Work out the finished part from the listing and answer in its coordinate system (mm). A direction names the side the tool comes from. Round coordinates to 2 decimals unless told otherwise and drop trailing zeros. Loops run counter-clockwise (first coordinate to the right, second up) from the corner with the lowest first, then second, coordinate; pieces in that order, holes last. Notation, with made-up numbers: M 8,11 L 57,11 A22 cw 57,41 Z; hole C 53.5,-9.5 d8. An arc over 180 degrees is marked long. One line per item, written item: value.
```python
from build123d import *

# Parameters (mm, degrees)
ESQUISSE1_W      = 31.5
ESQUISSE1_H      = 19
EXTRUSION1_DEPTH = 3
EXTRUSION2_DEPTH = 5


with BuildPart() as part:
    # Esquisse1 → Extrusion1 (new body)
    with BuildSketch(Plane.XY):
        with Locations((-6.993175074, -6.195994065)):
            Rectangle(ESQUISSE1_W, ESQUISSE1_H)
    extrude(amount=-EXTRUSION1_DEPTH)

    # Esquisse2 → Extrusion2 (add, symmetric)
    with BuildSketch(Plane(origin=(0, -6.445994065, 0), x_dir=(-1, 0, 0), z_dir=(0, 1, 0))):
        with BuildLine():
            Line((-0.683946914, 1.503708235), (-1.522862282, 2.753870501))
            Line((-1.522862282, 2.753870501), (-0.951110198, 2.753870501))
            Line((-0.951110198, 2.753870501), (-1.764464322, 4.339195483))
            Line((-1.764464322, 4.339195483), (-1.070373593, 4.339195483))
            Line((-1.070373593, 4.339195483), (-1.522862282, 6.137827556))
            Line((-1.522862282, 6.137827556), (-0.919586302, 6.039619438))
            Line((-0.919586302, 6.039619438), (-0.919586302, 7.896542483))
            Line((-0.919586302, 7.896542483), (-0.491311221, 7.750686861))
            Line((-0.491311221, 7.750686861), (-0.194631359, 9.573141446))
            Line((-0.194631359, 9.573141446), (0.23155106, 9.427998511))
            Line((0.23155106, 9.427998511), (0.646902561, 11.526197473))
            Line((0.646902561, 11.526197473), (-0.919586302, 12.794183433))
            ThreePointArc((-0.919586302, 12.794183433), (-1.739109574, 14.422451612), (0.024155253, 13.960095898))
            Line((0.024155253, 13.960095898), (1.735137514, 12.575150538))
            Line((1.735137514, 12.575150538), (3.580381554, 13.110240468))
            ThreePointArc((3.580381554, 13.110240468), (6.259156873, 14.419297059), (9.196563315, 14.930286061))
            ThreePointArc((9.196563315, 14.930286061), (16.439211341, 8.707680897), (11.226331582, 0.70751527))
            ThreePointArc((11.226331582, 0.70751527), (10.958201165, 0.354142581), (11.225313893, 0))
            Line((11.225313893, 0), (3.908893256, 0))
            ThreePointArc((3.908893256, 0), (4.942460115, 0.812425826), (4.628744056, 2.089092739))
            ThreePointArc((4.628744056, 2.089092739), (2.440830828, 5.172896926), (2.103130606, 8.938898932))
            ThreePointArc((2.103130606, 8.938898932), (2.971882266, 9.547397538), (3.580380872, 8.678645878))
            ThreePointArc((3.580380872, 8.678645878), (12.939531774, 3.276526542), (9.243174696, 13.431010442))
            ThreePointArc((9.243174696, 13.431010442), (1.988346124, 9.431080483), (0.985709709, 1.207535171))
            ThreePointArc((0.985709709, 1.207535171), (0.089542016, 1.009824881), (-0.683946914, 1.503708235))
        make_face()
        with BuildLine():
            Line((0.024155253, 9.573141446), (-0.573596034, 9.77671478))
            Line((-0.573596034, 9.77671478), (-3.903205639, 0))
            Line((-3.903205639, 0), (-5.477057205, 0))
            Line((-5.477057205, 0), (-2.145067788, 9.78370261))
            Line((-2.145067788, 9.78370261), (-5.43013268, 10.902481655))
            ThreePointArc((-5.43013268, 10.902481655), (-6.770419213, 12.151238044), (-4.946559165, 12.322395968))
            Line((-4.946559165, 12.322395968), (-0.453501716, 10.7922166))
            Line((-0.453501716, 10.7922166), (0.024155253, 9.573141446))
        make_face()
    extrude(amount=EXTRUSION2_DEPTH, both=True)


solid = part.part
```
1) Find section B-B (z = 6.75). Give the vertices of the cut face in (x, y).
Check values:
outline: M -16.45,-11.45 L -14.92,-11.45 L -14.92,-1.45 L -16.45,-1.45 Z; M -3.57,-11.45 L -2.05,-11.45 L -2.05,-1.45 L -3.57,-1.45 Z; M -0.75,-11.45 L 0.92,-11.45 L 0.92,-1.45 L -0.75,-1.45 Z; M 1.6,-11.45 L 3.18,-11.45 L 3.18,-1.45 L 1.6,-1.45 Z
2) Each of these flat-tipped pins is pushed along its axis until it touches: pin 1 (1.5 mm diameter, centred on x = -0.5, z = 3.5, fed in from +Y); pin 2 (4 mm diameter, centred on y = -5.5, z = 3, fed in from -X); pin 3 (10 mm diameter, centred on x = -17, y = -5, fed in from +Z). Where does it stop, or does it pass through?
Check values:
pin 1: y = -1.45
pin 2: x = -16
pin 3: z = 14.39
3) Find section C-C (x = -8). Give the vertices of the cut face in (y, z).
Check values:
outline: M -15.7,-3 L 3.3,-3 L 3.3,0 L -1.45,0 L -1.45,2.07 L -11.45,2.07 L -11.45,0 L -15.7,0 Z; M -11.45,13.31 L -1.45,13.31 L -1.45,14.82 L -11.45,14.82 Z
4) The mould has two halves that part along X. Classify faces 6 (the face through (-22.743, -6, -1)), 7 (the face through (1.759, -6.516, 14.397)), 8 (the face through (-3, -11.446, 8)): +X half, -X half, draft (parallel to the pull), parting line (faces both ways), or undercut.
Check values:
face 6: -X half
face 7: undercut
face 8: draft
5) Find section A-A (x = 2.5). Give the vertices of the cut face in (y, z), then the cut area to 3 significant figures.
Check values:
outline: M -15.7,-3 L 3.3,-3 L 3.3,0 L -15.7,0 Z; M -11.45,4.12 L -1.45,4.12 L -1.45,8.74 L -11.45,8.74 Z; M -11.45,9.9 L -1.45,9.9 L -1.45,11.49 L -11.45,11.49 Z
area: 119 mm2
6) Find the intervals of material crossed by probe 1 along X at (y, z) = (-2.5, 7); probe 2 along X at (y, z) = (-10, 7.5); probe 3 along Z at (x, y) = (-19.5, -4), in increasing order. Write a range as from..to.
Check values:
probe 1: -16.48..-14.95, -3.53..-2.03, -0.83..0.92, 1.52..3.09
probe 2: -16.51..-14.99, -3.5..-2, -1..0.92, 1.35..2.92
probe 3: -3..0
7) For faces 1 (the face through (2.6, -1.446, 6.9)), 2 (the face through (8.757, -6, -1)), 3 (the face through (-0.1, -6.52, 1.01)), 4 (the face through (3.834, -6.376, 4.823)), 5 (the face through (-2.645, -6.516, 12.839)), determine the directions among +Z, -Z, +X, -X, +Y, -Y from which every point of the face is accessible in a straight line to the end or side of a thin tool.
Check values:
face 1: +Z, +X, -X, +Y
face 2: +Z, -Z, +X, +Y, -Y
face 3: +Y, -Y
face 4: +X, +Y, -Y
face 5: +Z, +Y, -Y
8) Find section D-D (y = -13). Give the vertices of the cut face in (x, z), then the cut area to 3 significant figures.
Check values:
outline: M -22.74,-3 L 8.76,-3 L 8.76,0 L -22.74,0 Z
area: 94.5 mm2
